Could you check a few things on this model? Use its own coordinates, in mm. A direction names the side the tool comes from. Round coordinates to 2 decimals unless told otherwise and drop trailing zeros. Write each loop counter-clockwise with the first axis right and the second up, starting at its lowest first coordinate (ties: lowest second). Pieces come first, ordered by that corner, then holes. Notation, with made-up numbers: (-34, 2.25) -> (-27, 2.25) arc R21 cw to (-27, 31.25) -> close; hole circle Ø3 at (-16.75, 30.25). An arc over 180 degrees is marked (long way). Return JSON: item names as keys, results as strings.
from build123d import *

# Parameters (mm, degrees)
F1_DEPTH = 8.8
F2_DEPTH = 1
F3_R     = 2.5
F5_DEPTH = 4


with BuildPart() as f1:
    # F0 (on Top) → F1 (new body)
    with BuildSketch(Plane.XY):
        with BuildLine():
            ThreePointArc((-2.5, 0), (0, -2.5), (2.5, 0))
            ThreePointArc((2.5, 0), (0, 2.5), (-2.5, 0))
        make_face()
    extrude(amount=F1_DEPTH)

    # F0 (on Top) → F2 (join)
    with BuildSketch(Plane.XY):
        with BuildLine():
            Line((-2.5, 1.4197270865), (-2.5, 0))
            Line((-2.5, 0), (-2.5, -1.4197270865))
            ThreePointArc((-2.5, -1.4197270865), (2.875, 0), (-2.5, 1.4197270865))
        make_face()
        with BuildLine():
            ThreePointArc((-2.5, 0), (0, 2.5), (2.5, 0))
            ThreePointArc((2.5, 0), (0, -2.5), (-2.5, 0))
        make_face(mode=Mode.SUBTRACT)
        with BuildLine():
            ThreePointArc((-2.5, 0), (0, -2.5), (2.5, 0))
            ThreePointArc((2.5, 0), (0, 2.5), (-2.5, 0))
        make_face()
    extrude(amount=F2_DEPTH)

    # F3
    f3_edges = [f1.edges().sort_by_distance(p)[0] for p in [
        (-2.5, 0, 8.8),
    ]]
    fillet(f3_edges, radius=F3_R)

    # F4 (on face) → F5 (join)
    with BuildSketch(Plane(origin=(0, 0, 0), x_dir=(1, 0, 0), z_dir=(0, 0, -1))):
        Polygon((1, 0.25), (1, 0), (1, -0.25), (1.5, -0.25), (1.5, 0.25), align=None)
        Polygon((-1, 0.25), (-1.5, 0.25), (-1.5, -0.25), (-1, -0.25), (-1, 0), align=None)
    extrude(amount=F5_DEPTH)


solid = f1.part
1) I want a section at C-C, the plane y = -0.7. Please give me the cut outline in (x, z), and give its area (3 significant figures).
Return value:
{"outline": "(-2.5, 0) -> (2.79, 0) -> (2.79, 1) -> (2.4, 1) -> (2.4, 6.3) arc R2.4 ccw to (-2.4, 6.3) -> (-2.4, 1) -> (-2.5, 1) -> close", "area": "39.8 mm²"}
2) Will these pins go through, and if not, where does the flat tip stop? pin 1 Ø2.5 at (x, y) = (-0.5, 1.5) entering from -Z; pin 2 Ø1 at (x, z) = (-1.5, -1) entering from -Y; pin 3 Ø0.6 at (x, z) = (1.5, -2.5) entering from +Y.
Return value:
{"pin 1": "z = 0", "pin 2": "y = -0.25", "pin 3": "y = 0.25"}
3) I want a section at D-D, the plane z = 2.75. Please give me the cut outline in (x, y).
Return value:
{"outline": "circle Ø5 at (0, 0)"}
4) If I drill on probe 1 along Z at (x, y) = (-2.2, 1.55); probe 2 along X at (y, z) = (-0.65, 3.25); probe 3 along X at (y, z) = (1, 4.25), over which ranges is the centre line in solid material (lowest first)? Write a range as [from, to].
Return value:
{"probe 1": "[0, 1]", "probe 2": "[-2.41, 2.41]", "probe 3": "[-2.29, 2.29]"}
5) For faces 1 (the face through (-2, -1.5, 3.6)), 2 (the face through (2.873, -0.106, 0.493)), which set-ups out of +Z, -Z, +X, -X, +Y, -Y let a thin tool reach every point of the face, with its end or its side?
Return value:
{"face 1": "+Z", "face 2": "+Z, -Z"}
6) I want a section at A-A, the plane z = -1. Please give me the cut outline in (x, y).
Return value:
{"outline": "(-1.5, -0.25) -> (-1, -0.25) -> (-1, 0.25) -> (-1.5, 0.25) -> close; (1, -0.25) -> (1.5, -0.25) -> (1.5, 0.25) -> (1, 0.25) -> close"}
7) I want a section at B-B, the plane x = 0. Please give me the cut outline in (y, z) (3 decimals), and give its area (3 significant figures).
Return value:
{"outline": "(-2.875, 0) -> (2.875, 0) -> (2.875, 1) -> (2.5, 1) -> (2.5, 6.3) arc R2.5 ccw to (-2.5, 6.3) -> (-2.5, 1) -> (-2.875, 1) -> close", "area": "42.1 mm²"}
